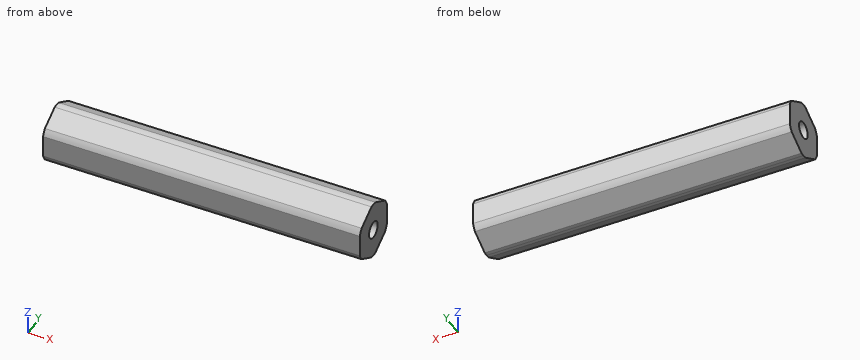
from build123d import *

# Parameters (mm, degrees)
SKETCH1_R           = 2.0193
BOSS_EXTRUDE1_DEPTH = 38.1


with BuildPart() as part:
    # Sketch1 → Boss-Extrude1 (new, symmetric)
    with BuildSketch(Plane(origin=(0, 0, 0), x_dir=(0, 0, -1), z_dir=(1, 0, 0))):
        with BuildLine():
            ThreePointArc((6.874999966, 0), (6.860422465, 0.447468582), (6.816751782, 0.893039571))
            Line((6.816751782, 0.893039571), (4.181770846, 5.456960429))
            ThreePointArc((4.181770846, 5.456960429), (3.437499983, 5.953924622), (2.634980936, 6.35))
            Line((2.634980936, 6.35), (-2.634980936, 6.35))
            ThreePointArc((-2.634980936, 6.35), (-3.437499983, 5.953924622), (-4.181770846, 5.456960429))
            Line((-4.181770846, 5.456960429), (-6.816751782, 0.893039571))
            ThreePointArc((-6.816751782, 0.893039571), (-6.874999966, 0), (-6.816751782, -0.893039571))
            Line((-6.816751782, -0.893039571), (-4.181770846, -5.456960429))
            ThreePointArc((-4.181770846, -5.456960429), (-3.437499983, -5.953924622), (-2.634980936, -6.35))
            Line((-2.634980936, -6.35), (2.634980936, -6.35))
            ThreePointArc((2.634980936, -6.35), (3.437499983, -5.953924622), (4.181770846, -5.456960429))
            Line((4.181770846, -5.456960429), (6.816751782, -0.893039571))
            ThreePointArc((6.816751782, -0.893039571), (6.860422465, -0.447468582), (6.874999966, 0))
        make_face()
        Circle(SKETCH1_R, mode=Mode.SUBTRACT)
    extrude(amount=BOSS_EXTRUDE1_DEPTH, both=True)


solid = part.part
The listing builds one solid part. Answer for the finished solid, in the listing's coordinates (mm). Give positions to 0.01 mm unless a question says otherwise; leave off trailing zeros. Write each loop counter-clockwise with the first axis right and the second up, starting at its lowest first coordinate (ties: lowest second). Pieces come first, ordered by that corner, then holes.
1) Section C-C (y = 3.25) is taken. Write down the section's boundary in (x, z), and give its area (3 significant figures).
2) Section A-A (z = 0) is taken. Write down the section's boundary in (x, y).
3) Given P1, Ø1.5, axis at x = 15.5, z = -4.5, coming from the +Y side; P2, Ø3, axis at x = -23.5, y = -2.5, coming from the +Z side (3 decimals); P3, Ø4, axis at x = 5, y = -3, coming from the -Z side (3 decimals); P4, Ø4, axis at x = -24, z = -4.5, coming from the +Y side, each flat-ended and moving along its own axis, determine where each tip first touches the part or whether it passes through.
4) Find the intervals of material crossed by L1, parallel to Y at x = -4.5, z = 0; L2, parallel to Z at x = -30.5, y = 3.25; L3, parallel to Y at x = 18, z = -1.5, in increasing order.
5) Section B-B (x = 9.5) is taken. Write down the section's boundary in (y, z) (3 decimals), and give its area (3 significant figures).
6) Section D-D (z = 5.5) is taken. Write down the section's boundary in (x, y), and give its area (3 significant figures).
Response:
1. outline: (-38.1, -5.46) - (38.1, -5.46) - (38.1, 5.46) - (-38.1, 5.46) - close
1. area: 831 mm2
2. outline: (-38.1, -6.35) - (38.1, -6.35) - (38.1, -2.02) - (-38.1, -2.02) - close; (-38.1, 2.02) - (38.1, 2.02) - (38.1, 6.35) - (-38.1, 6.35) - close
3. P1: stops at y = 5.76
3. P2: stops at z = 6.755
3. P3: stops at z = -6.755
3. P4: stops at y = 6.35
4. L1: y = -6.35 to -2.02, 2.02 to 6.35
4. L2: z = -5.46 to 5.46
4. L3: y = -6.35 to -1.35, 1.35 to 6.35
5. outline: (-6.35, -2.635) arc R6.875 ccw to (-5.457, -4.182) - (-0.893, -6.817) arc R6.875 ccw to (0.893, -6.817) - (5.457, -4.182) arc R6.875 ccw to (6.35, -2.635) - (6.35, 2.635) arc R6.875 ccw to (5.457, 4.182) - (0.893, 6.817) arc R6.875 ccw to (-0.893, 6.817) - (-5.457, 4.182) arc R6.875 ccw to (-6.35, 2.635) - close; hole circle Ø4.039 at (0, 0)
5. area: 125 mm2
6. outline: (-38.1, -3.17) - (38.1, -3.17) - (38.1, 3.17) - (-38.1, 3.17) - close
6. area: 484 mm2
